Design review of the part built by this model. Coordinates are the model's own, in mm. A direction names the side the tool comes from. Give positions to 0.01 mm unless a question says otherwise; leave off trailing zeros. Loops run counter-clockwise (first coordinate to the right, second up) from the corner with the lowest first, then second, coordinate; pieces in that order, holes last.
from build123d import *

# Parameters (mm, degrees)
SKETCH_W        = 60
SKETCH_H        = 80
PAD_DEPTH       = 10
SKETCH001_W     = 56
SKETCH001_H     = 76
POCKET_DEPTH    = 2
SKETCH002_W     = 20
SKETCH002_H     = 35.5
SKETCH002_W_2   = 45
SKETCH002_H_2   = 30
SKETCH002_W_3   = 7.5
SKETCH002_H_3   = 35
POCKET001_DEPTH = 6
SKETCH003_W     = 14
SKETCH003_H     = 6
POCKET002_DEPTH = 5
FILLET_R        = 3
SKETCH004_R     = 1.75
POCKET003_DEPTH = 10
POCKET004_DEPTH = 6
SKETCH013_W     = 10
SKETCH013_H     = 10
POCKET011_DEPTH = 6


with BuildPart() as part:
    # Sketch → Pad (new body)
    with BuildSketch(Plane.XY):
        Rectangle(SKETCH_W, SKETCH_H)
    extrude(amount=PAD_DEPTH)

    # Sketch001 (on Face6 of Pad) → Pocket (cut)
    with BuildSketch(Plane.XY.offset(10)):
        Rectangle(SKETCH001_W, SKETCH001_H)
    extrude(amount=-POCKET_DEPTH, mode=Mode.SUBTRACT)

    # Sketch002 (on Face11 of Pocket) → Pocket001 (cut)
    with BuildSketch(Plane.XY.offset(8)):
        with Locations((0, 20.25)):
            Rectangle(SKETCH002_W, SKETCH002_H)
        with Locations((0, -17.5)):
            Rectangle(SKETCH002_W_2, SKETCH002_H_2)
        with Locations((-18.75, 15)):
            Rectangle(SKETCH002_W_3, SKETCH002_H_3)
        with Locations((18.75, 15)):
            Rectangle(SKETCH002_W_3, SKETCH002_H_3)
    extrude(amount=-POCKET001_DEPTH, mode=Mode.SUBTRACT)

    # Sketch003 (on Face24 of Pocket001) → Pocket002 (cut)
    with BuildSketch(Plane.XZ.offset(-38)):
        with Locations((0, 5)):
            Rectangle(SKETCH003_W, SKETCH003_H)
    extrude(amount=-POCKET002_DEPTH, mode=Mode.SUBTRACT)

    # Fillet
    fillet_edges = [part.edges().sort_by_distance(p)[0] for p in [
        (-30, -40, 5),
        (-30, 40, 5),
        (30, -40, 5),
        (30, 40, 5),
    ]]
    fillet(fillet_edges, radius=FILLET_R)

    # Sketch004 (on Face19 of Fillet) → Pocket003 (cut)
    with BuildSketch(Plane.XY.offset(8)):
        with Locations((26, -36)):
            Circle(SKETCH004_R)
        with Locations((-26, -36)):
            Circle(SKETCH004_R)
        with Locations((-26, 36)):
            Circle(SKETCH004_R)
        with Locations((26, 36)):
            Circle(SKETCH004_R)
    extrude(amount=-POCKET003_DEPTH, mode=Mode.SUBTRACT)

    # Sketch005 (on Face2 of Pocket003) → Pocket004 (cut)
    with BuildSketch(Plane(origin=(0, 0, 0), x_dir=(1, 0, 0), z_dir=(0, 0, -1))):
        Polygon((-24.375, 33.185417), (-22.75, 36), (-24.375, 38.814583), (-27.625, 38.814583), (-29.25, 36), (-27.625, 33.185417), align=None)
        Polygon((27.625, 33.185417), (29.25, 36), (27.625, 38.814583), (24.375, 38.814583), (22.75, 36), (24.375, 33.185417), align=None)
        Polygon((-22.75, -36), (-24.375, -33.185417), (-27.625, -33.185417), (-29.25, -36), (-27.625, -38.814583), (-24.375, -38.814583), align=None)
        Polygon((29.25, -36), (27.625, -33.185417), (24.375, -33.185417), (22.75, -36), (24.375, -38.814583), (27.625, -38.814583), align=None)
    extrude(amount=-POCKET004_DEPTH, mode=Mode.SUBTRACT)

    # Sketch013 (on Face47 of Pocket004) → Pocket011 (cut)
    with BuildSketch(Plane.XY.offset(8)):
        Rectangle(SKETCH013_W, SKETCH013_H)
    extrude(amount=-POCKET011_DEPTH, mode=Mode.SUBTRACT)


solid = part.part
Q1. Take a section at A-A (z = 7). Give the number of separate pieces and of enclosed holes in the cut face, plus the area to 3 significant figures.
Results:
separate pieces: 1
enclosed holes: 4
area: 2,090 mm2
Q2. Draft analysis for pull direction X (two halves, no side actions). For faces 1 (the face through (-30, -1, 5)), 2 (the face through (0, -40, 5)), 3 (the face through (24.61, -37.06, 7.01)), state which applies: pulls with the +X half, pulls with the -X half, needs draft (parallel to the pull), parting line crosses it, or undercut.
Results:
face 1: pulls with the -X half
face 2: needs draft
face 3: undercut
Q3. Tool access review of faces 4 (the face through (15, 15, 5)), 5 (the face through (-26, -38.815, 3)), 6 (the face through (-0.4, 40, 1.6)): name each direction out of +Z, -Z, +X, -X, +Y, -Y from which nothing blocks a thin tool from reaching the whole face with its end or side.
Results:
face 4: +Z
face 5: -Z
face 6: +Z, -Z, +X, -X, +Y
Q4. Insertion check: pin 1 (1.6 mm diameter, centred on y = 39.5, z = 5.5, fed in from +X); pin 2 (1.7 mm diameter, centred on x = -25.5, y = -37.5, fed in from -Z); pin 3 (3 mm diameter, centred on x = -26, y = 36, fed in from -Z). Each pin has a flat end and moves straight along its axis. Give the tip position at first contact, or say it passes through.
Results:
pin 1: stops at x = 29.47
pin 2: stops at z = 6
pin 3: passes through
Q5. Take a section at D-D (y = -23). Give the boundary of the cut face in (x, z), plus the area to 3 significant figures.
Results:
outline: (-30, 0) - (30, 0) - (30, 10) - (28, 10) - (28, 8) - (22.5, 8) - (22.5, 2) - (-22.5, 2) - (-22.5, 8) - (-28, 8) - (-28, 10) - (-30, 10) - close
area: 218 mm2
Q6. Wall thickness on line 1 (Y direction, x = -26, z = 7.4); line 2 (X direction, y = 28.5, z = 4.5); line 3 (Y direction, x = 9, z = 7.25): over which ranges is each line inside the solid? List them lowest first.
Results:
line 1: y = -40 to -37.75, -34.25 to 34.25, 37.75 to 40
line 2: x = -30 to -22.5, -15 to -10, 10 to 15, 22.5 to 30
line 3: y = -40 to -32.5, -2.5 to 2.5, 38 to 40
Q7. Take a section at C-C (y = 4). Give the boundary of the cut face in (x, z).
Results:
outline: (-30, 0) - (30, 0) - (30, 10) - (28, 10) - (28, 8) - (22.5, 8) - (22.5, 2) - (15, 2) - (15, 8) - (10, 8) - (10, 2) - (-10, 2) - (-10, 8) - (-15, 8) - (-15, 2) - (-22.5, 2) - (-22.5, 8) - (-28, 8) - (-28, 10) - (-30, 10) - close
Q8. Take a section at B-B (x = 26). Give the boundary of the cut face in (y, z), plus the area to 3 significant figures.
Results:
outline: (-40, 0) - (-38.81, 0) - (-38.81, 6) - (-37.75, 6) - (-37.75, 8) - (-38, 8) - (-38, 10) - (-40, 10) - close; (-34.25, 6) - (-33.19, 6) - (-33.19, 0) - (33.19, 0) - (33.19, 6) - (34.25, 6) - (34.25, 8) - (-34.25, 8) - close; (37.75, 6) - (38.81, 6) - (38.81, 0) - (40, 0) - (40, 10) - (38, 10) - (38, 8) - (37.75, 8) - close
area: 566 mm2
